The listing builds one solid part. Answer for the finished solid, in the listing's coordinates (mm). A direction names the side the tool comes from. Round coordinates to 2 decimals unless told otherwise and drop trailing zeros. Write each loop counter-clockwise with the first axis right and the second up, starting at its lowest first coordinate (ties: lowest second). Pieces come first, ordered by that corner, then holes. Notation, with made-up numbers: (6, -20) - (46, -20) arc R6 cw to (46, -9) - close; hole circle Ø8 at (66.5, 2). An arc over 180 degrees is marked (long way). Answer in a Markdown table with one row per item.
from build123d import *

# Parameters (mm, degrees)
BOSS_EXTRUDE1_DEPTH     = 3
FILLET2_R               = 4
SKETCH7_R               = 1.6
CUT_EXTRUDE2_DEPTH      = 1
CUT_EXTRUDE2_DEPTH_BACK = 4
SKETCH4_W               = 44
SKETCH4_H               = 94
CUT_EXTRUDE3_DEPTH      = 10
FILLET3_R               = 1.5


with BuildPart() as part:
    # Sketch3 → Boss-Extrude1 (new body)
    with BuildSketch(Plane(origin=(0, 0, 0), x_dir=(1, 0, 0), z_dir=(0, 1, 0))):
        Polygon((70, 80), (-22, 80), (-22, 35), (-50, 35), (-50, -15), (-22, -15), (-22, -60), (70, -60), (70, -12.5), (42, -12.5), (42, 32.5), (70, 32.5), align=None)
    extrude(amount=BOSS_EXTRUDE1_DEPTH)

    # Fillet2
    fillet2_edges = [part.edges().sort_by_distance(p)[0] for p in [
        (70, 1.5, 12.5),
        (70, 1.5, 60),
        (-22, 1.5, 60),
        (-50, 1.5, 15),
        (-50, 1.5, -35),
        (-22, 1.5, -80),
        (70, 1.5, -80),
        (70, 1.5, -32.5),
    ]]
    fillet(fillet2_edges, radius=FILLET2_R)

    # Sketch7 → Cut-Extrude2 (cut, two sides)
    with BuildSketch(Plane(origin=(0, 3, 0), x_dir=(1, 0, 0), z_dir=(0, 1, 0))) as cut_extrude2_sk:
        with Locations((-46, 31)):
            Circle(SKETCH7_R)
        with Locations((-46, -11)):
            Circle(SKETCH7_R)
        with Locations((66, -56)):
            Circle(SKETCH7_R)
        with Locations((66, 76)):
            Circle(SKETCH7_R)
        with Locations((-10, 76)):
            Circle(SKETCH7_R)
        with Locations((-10, -56)):
            Circle(SKETCH7_R)
        with Locations((30, -56)):
            Circle(SKETCH7_R)
        with Locations((30, 76)):
            Circle(SKETCH7_R)
        with Locations((66, -16.5)):
            Circle(SKETCH7_R)
        with Locations((66, 36.5)):
            Circle(SKETCH7_R)
    extrude(amount=CUT_EXTRUDE2_DEPTH, mode=Mode.SUBTRACT)
    extrude(cut_extrude2_sk.sketch, amount=-CUT_EXTRUDE2_DEPTH_BACK, mode=Mode.SUBTRACT)

    # Sketch4 → Cut-Extrude3 (cut)
    with BuildSketch(Plane(origin=(0, 3, 0), x_dir=(1, 0, 0), z_dir=(0, 1, 0))):
        with Locations((10, 10)):
            Rectangle(SKETCH4_W, SKETCH4_H)
    extrude(amount=-CUT_EXTRUDE3_DEPTH, mode=Mode.SUBTRACT)

    # Fillet3
    fillet3_edges = [part.edges().sort_by_distance(p)[0] for p in [
        (32, 1.5, -57),
        (32, 1.5, 37),
        (-12, 1.5, 37),
        (-12, 1.5, -57),
        (-22, 0, 35.5),
        (-34, 0, -35),
        (54, 0, -32.5),
        (42, 0, -10),
        (42, 1.5, 12.5),
        (-22, 1.5, 15),
        (-22, 1.5, -35),
        (42, 1.5, -32.5),
        (-22, 0, -55.5),
        (54, 0, 12.5),
        (70, 0, 36.25),
        (24, 0, 60),
        (-34, 0, 15),
        (-50, 0, -10),
        (24, 0, -80),
        (70, 0, -56.25),
        (68.828427125, 0, 58.828427125),
        (68.828427125, 0, 13.671572875),
        (-20.828427125, 0, 58.828427125),
        (-48.828427125, 0, 13.828427125),
        (-48.828427125, 0, -33.828427125),
        (68.828427125, 0, -78.828427125),
        (68.828427125, 0, -33.671572875),
        (-20.828427125, 0, -78.828427125),
    ]]
    fillet(fillet3_edges, radius=FILLET3_R)


solid = part.part
(1) Find the intervals of material crossed by line 1 (Z direction, x = -10, y = 2.2); line 2 (X direction, y = 2.35, z = -76); line 3 (Z direction, x = 66, y = 2.15), in increasing order.
Checked values:
| item | result |
|---|---|
| line 1 | z = -80 to -77.6, -74.4 to -57, 37 to 54.4, 57.6 to 60 |
| line 2 | x = -22 to -11.6, -8.4 to 28.4, 31.6 to 64.4, 67.6 to 70 |
| line 3 | z = -80 to -77.6, -74.4 to -38.1, -34.9 to -32.5, 12.5 to 14.9, 18.1 to 54.4, 57.6 to 60 |
(2) Section B-B (x = 7.5) is taken. Give the vertices of the cut face in (y, z).
Checked values:
| item | result |
|---|---|
| outline | (0, -78.5) arc R1.5 ccw to (1.5, -80) - (3, -80) - (3, -57) - (0, -57) - close; (0, 37) - (3, 37) - (3, 60) - (1.5, 60) arc R1.5 ccw to (0, 58.5) - close |
(3) For faces 4 (the cylindrical face through (-48.797, 2.26, -33.859)), 5 (the cylindrical face through (68.797, 2.26, -33.641)), 6 (the flat face through (10, 2, 37)), determine the directions among +Z, -Z, +X, -X, +Y, -Y from which every point of the face is accessible in a straight line to the end or side of a thin tool.
Checked values:
| item | result |
|---|---|
| face 4 | -Z, -X, +Y, -Y |
| face 5 | +X, +Y, -Y |
| face 6 | +Y, -Y |
(4) Flat-ended cylindrical pins translate along their axes: pin 1 (1.2 mm diameter, centred on y = 2, z = -65, fed in from -X); pin 2 (0.8 mm diameter, centred on x = -33, y = 2, fed in from -Z); pin 3 (1.7 mm diameter, centred on x = -32, y = 2.5, fed in from +Z); pin 4 (5 mm diameter, centred on x = 66, z = 16.5, fed in from +Y). Find the tip coordinate at first contact, or state that the pin passes through.
Checked values:
| item | result |
|---|---|
| pin 1 | stops at x = -22 |
| pin 2 | stops at z = -35 |
| pin 3 | stops at z = 15 |
| pin 4 | stops at y = 3 |
(5) Section A-A (z = -23) is taken. Give the vertices of the cut face in (x, y), and give its area (3 significant figures).
Checked values:
| item | result |
|---|---|
| outline | (-50, 1.5) arc R1.5 ccw to (-48.5, 0) - (-12, 0) - (-12, 3) - (-50, 3) - close; (32, 0) - (40.5, 0) arc R1.5 ccw to (42, 1.5) - (42, 3) - (32, 3) - close |
| area | 143 mm2 |
(6) Section C-C (y = 2) is taken. State how many separate pieces and enclosed holes the cut face has, and give its area (3 significant figures).
Checked values:
| item | result |
|---|---|
| separate pieces | 1 |
| enclosed holes | 11 |
| area | 8,780 mm2 |
(7) For a pull along Z with two mould halves and no side action, classify faces 1 (the cylindrical face through (-20.859, 2.26, 58.797)), 2 (the cylindrical face through (68.797, 2.26, -78.859)), 3 (the cylindrical face through (-11.6, 1.52, -76.07)) as pulls with the +Z half, pulls with the -Z half, needs draft (parallel to the pull), parting line crosses it, or undercut.
Checked values:
| item | result |
|---|---|
| face 1 | pulls with the +Z half |
| face 2 | pulls with the -Z half |
| face 3 | undercut |
(8) Section D-D (x = -30) is taken. Give the vertices of the cut face in (y, z).
Checked values:
| item | result |
|---|---|
| outline | (0, -33.5) arc R1.5 ccw to (1.5, -35) - (3, -35) - (3, 15) - (1.5, 15) arc R1.5 ccw to (0, 13.5) - close |
